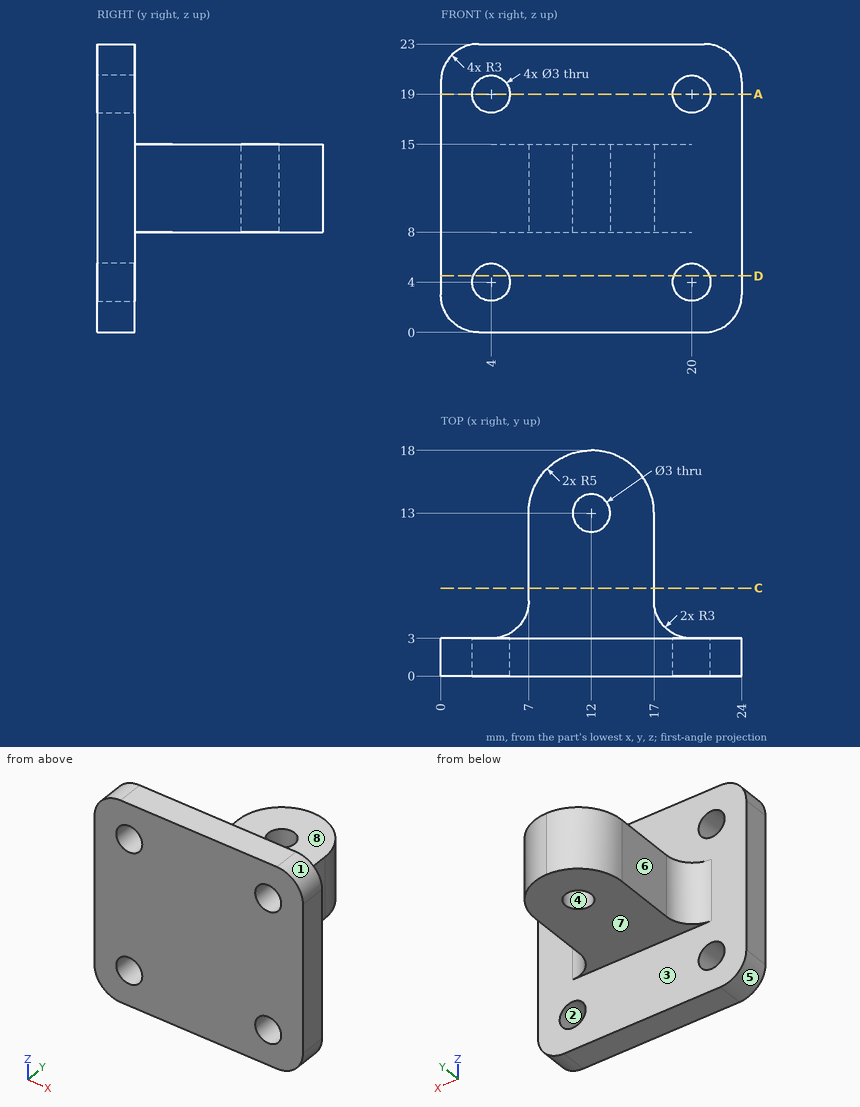
Could you check a few things on this drawing? It's one solid part, dimensions in mm from its lowest x, y, z. A direction names the side the tool comes from. Give positions to 0.01 mm unless a question says otherwise; leave off trailing zeros. Loops run counter-clockwise (first coordinate to the right, second up) from the corner with the lowest first, then second, coordinate; pieces in that order, holes last. Notation, with made-up numbers: M 41.25,56 L 90.25,56 A13 ccw 90.25,69 Z; hole C -39,30 d9. An arc over 180 degrees is marked long. Answer as a JSON object with one key per item and string values.
Q1. If I drill on probe 1 along X at (y, z) = (1.5, 19); probe 2 along Y at (x, z) = (10.75, 20); probe 3 along X at (y, z) = (9.25, 10.5), over which ranges is the centre line in solid material (lowest first)? Write a range as [from, to].
Values found:
{"probe 1": "x = [0, 2.5], [5.5, 18.5], [21.5, 24]", "probe 2": "y = [0, 3]", "probe 3": "x = [7, 17]"}
Q2. Suppose I cut it at A-A, the plane z = 19. List the corners of the cut face in (x, y) for me, plus the area to 3 significant figures.
Values found:
{"outline": "M 0,0 L 2.5,0 L 2.5,3 L 0,3 Z; M 5.5,0 L 18.5,0 L 18.5,3 L 5.5,3 Z; M 21.5,0 L 24,0 L 24,3 L 21.5,3 Z", "area": "54.0 mm²"}
Q3. Suppose I cut it at D-D, the plane z = 4.5. List the corners of the cut face in (x, y) for me.
Values found:
{"outline": "M 0,0 L 2.59,0 L 2.59,3 L 0,3 Z; M 5.41,0 L 18.59,0 L 18.59,3 L 5.41,3 Z; M 21.41,0 L 24,0 L 24,3 L 21.41,3 Z"}
Q4. For P1, Ø7.5, axis at y = 9, z = 11, coming from the +X side; P2, Ø10, axis at x = 12, z = 17, coming from the +Y side; P3, Ø6, axis at x = 11.5, y = 7.5, coming from the +Z side; P4, Ø1, axis at x = 14.5, y = 8.5, coming from the -Z side, each with a flat end and sliding along its axis, tell me the tip position at first contact or that it passes through.
Values found:
{"P1": "stops at x = 17.1", "P2": "stops at y = 18", "P3": "stops at z = 15", "P4": "stops at z = 8"}
Q5. For the marked faces 4, 5, 6, 7 and 8, which set-ups out of +Z, -Z, +X, -X, +Y, -Y let a thin tool reach every point of the face, with its end or its side?
Values found:
{"face 4": "+Z, -Z", "face 5": "-Z, -X, +Y, -Y", "face 6": "+Z, -Z, -X, +Y", "face 7": "-Z, +X, -X, +Y", "face 8": "+Z, +X, -X, +Y"}
Q6. Suppose I cut it at C-C, the plane y = 7. List the corners of the cut face in (x, z) for me, plus the area to 3 significant figures.
Values found:
{"outline": "M 7,8 L 17,8 L 17,15 L 7,15 Z", "area": "70.0 mm²"}
Q7. If we mould it in two halves opening along X, with no side actions, what happens to the marked faces 1, 2 and 3? For each: pulls with the +X half, pulls with the -X half, needs draft (parallel to the pull), parting line crosses it, or undercut.
Values found:
{"face 1": "pulls with the +X half", "face 2": "undercut", "face 3": "needs draft"}
